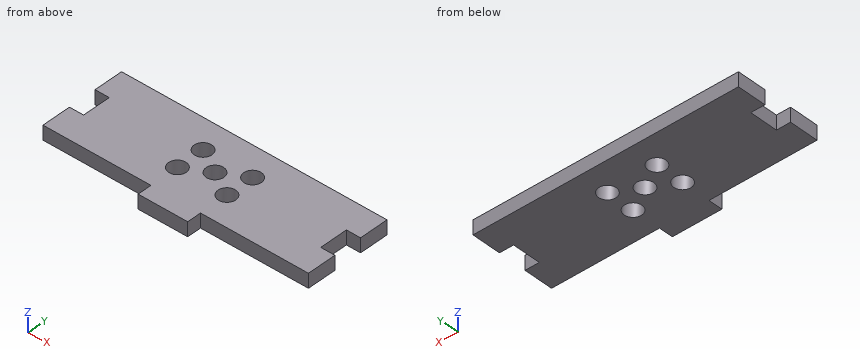
```python
from build123d import *

# Parameters (mm, degrees)
CROQUIS1_R              = 2.5
SALIENTE_EXTRUIR1_DEPTH = 4


with BuildPart() as part:
    # Croquis1 → Saliente-Extruir1 (new body)
    with BuildSketch(Plane.XY):
        Polygon((37.5, 12.25), (-37.5, 12.25), (-37.5, 4), (-33.5, 4), (-33.5, -4), (-37.5, -4), (-37.5, -12.25), (-7, -12.25), (-7, -16.25), (7, -16.25), (7, -12.25), (37.5, -12.25), (37.5, -4), (33.5, -4), (33.5, 4), (37.5, 4), align=None)
        Circle(CROQUIS1_R, mode=Mode.SUBTRACT)
        with Locations((7, 4)):
            Circle(CROQUIS1_R, mode=Mode.SUBTRACT)
        with Locations(Location((7, -4, 0), (0, 0, 180))):
            Circle(CROQUIS1_R, mode=Mode.SUBTRACT)
        with Locations((-7, -4)):
            Circle(CROQUIS1_R, mode=Mode.SUBTRACT)
        with Locations(Location((-7, 4, 0), (0, 0, 180))):
            Circle(CROQUIS1_R, mode=Mode.SUBTRACT)
    extrude(amount=SALIENTE_EXTRUIR1_DEPTH)


solid = part.part
```
Here's how the part is built. I have some questions about the finished solid (model axes, mm). Coordinates: 2 decimals unless noted, no trailing zeros. Order: outer loops, then holes, each group sorted by start corner. A loop starts at its lowest first (then second) coordinate and runs counter-clockwise, first axis right, second up.
1) Imagine slicing it at B-B on y = 0. List the corners of the cut face in (x, z) for me.
2) I need wall thicknesses on line 1 (X direction, y = -6, z = 2.4); line 2 (X direction, y = 2, z = 3.65); line 3 (X direction, y = 3.25, z = 3.7). Which ranges of each line are inside material? Lowest first, please.
3) Imagine slicing it at D-D on y = -4.75. List the corners of the cut face in (x, z) for me, and give its area (3 significant figures).
4) Will these pins go through, and if not, where does the flat tip stop? pin 1 (8 mm diameter, centred on x = -7, y = -4, fed in from -Z); pin 2 (1.2 mm diameter, centred on y = 1, z = 2, fed in from -X); pin 3 (1.5 mm diameter, centred on x = -23.5, z = 0.5, fed in from -Y).
5) Imagine slicing it at A-A on x = 0. List the corners of the cut face in (y, z) for me.
6) Imagine slicing it at C-C on z = 0.9. List the corners of the cut face in (x, y) for me.
Response values:
1. outline: (-33.5, 0) - (-2.5, 0) - (-2.5, 4) - (-33.5, 4) - close; (2.5, 0) - (33.5, 0) - (33.5, 4) - (2.5, 4) - close
2. line 1: x = -37.5 to -8.5, -5.5 to 5.5, 8.5 to 37.5
2. line 2: x = -33.5 to -8.5, -5.5 to -1.5, 1.5 to 5.5, 8.5 to 33.5
2. line 3: x = -33.5 to -9.38, -4.62 to 4.62, 9.38 to 33.5
3. outline: (-37.5, 0) - (-9.38, 0) - (-9.38, 4) - (-37.5, 4) - close; (-4.62, 0) - (4.62, 0) - (4.62, 4) - (-4.62, 4) - close; (9.38, 0) - (37.5, 0) - (37.5, 4) - (9.38, 4) - close
3. area: 262 mm2
4. pin 1: stops at z = 0
4. pin 2: stops at x = -33.5
4. pin 3: stops at y = -12.25
5. outline: (-16.25, 0) - (-2.5, 0) - (-2.5, 4) - (-16.25, 4) - close; (2.5, 0) - (12.25, 0) - (12.25, 4) - (2.5, 4) - close
6. outline: (-37.5, -12.25) - (-7, -12.25) - (-7, -16.25) - (7, -16.25) - (7, -12.25) - (37.5, -12.25) - (37.5, -4) - (33.5, -4) - (33.5, 4) - (37.5, 4) - (37.5, 12.25) - (-37.5, 12.25) - (-37.5, 4) - (-33.5, 4) - (-33.5, -4) - (-37.5, -4) - close; hole circle Ø5 at (-7, -4); hole circle Ø5 at (-7, 4); hole circle Ø5 at (0, 0); hole circle Ø5 at (7, -4); hole circle Ø5 at (7, 4)
